from build123d import *

# Parameters (mm, degrees)
F0_R     = 11.1
F1_DEPTH = 7.5
F0_R_2   = 4.25
F2_DEPTH = 7.5
F3_R     = 1.6
F4_DEPTH = 30.501
F5_SIZE  = 0.3
F6_DEPTH = 2.5


with BuildPart() as f1:
    # F0 (on Top) → F1 (new body)
    with BuildSketch(Plane.XY):
        with BuildLine():
            ThreePointArc((0, -14), (9.8994949366, -9.8994949366), (14, 0))
            ThreePointArc((14, 0), (9.8994949366, 9.8994949366), (0, 14))
            ThreePointArc((0, 14), (-14, 0), (0, -14))
        make_face()
        Circle(F0_R, mode=Mode.SUBTRACT)
        with BuildLine():
            ThreePointArc((0, 14), (9.8994949366, 9.8994949366), (14, 0))
            ThreePointArc((14, 0), (9.8994949366, -9.8994949366), (0, -14))
            Line((0, -14), (14, -14))
            Line((14, -14), (14, -22))
            Line((14, -22), (16.5, -22))
            Line((16.5, -22), (16.5, 0))
            Line((16.5, 0), (16.5, 22))
            Line((16.5, 22), (14, 22))
            Line((14, 22), (14, 14))
            Line((14, 14), (0, 14))
        make_face()
    extrude(amount=F1_DEPTH)

    # F0 (on Top) → F2 (join)
    with BuildSketch(Plane.XY):
        with BuildLine():
            ThreePointArc((0, 14), (9.8994949366, 9.8994949366), (14, 0))
            ThreePointArc((14, 0), (9.8994949366, -9.8994949366), (0, -14))
            Line((0, -14), (14, -14))
            Line((14, -14), (14, -22))
            Line((14, -22), (16.5, -22))
            Line((16.5, -22), (16.5, 0))
            Line((16.5, 0), (16.5, 22))
            Line((16.5, 22), (14, 22))
            Line((14, 22), (14, 14))
            Line((14, 14), (0, 14))
        make_face()
        with BuildLine():
            ThreePointArc((0, -14), (9.8994949366, -9.8994949366), (14, 0))
            ThreePointArc((14, 0), (9.8994949366, 9.8994949366), (0, 14))
            ThreePointArc((0, 14), (-14, 0), (0, -14))
        make_face()
        Circle(F0_R, mode=Mode.SUBTRACT)
        Circle(F0_R)
        Circle(F0_R_2, mode=Mode.SUBTRACT)
    extrude(amount=-F2_DEPTH)

    # F3 (on face) → F4 (cut, through all)
    with BuildSketch(Plane.YZ.offset(16.5)):
        with Locations((18, 0)):
            Circle(F3_R)
        with Locations((-18, 0)):
            Circle(F3_R)
    extrude(amount=-F4_DEPTH, mode=Mode.SUBTRACT)

    # F5
    f5_edges = [f1.edges().sort_by_distance(p)[0] for p in [
        (7, -14, -7.5),
        (14, -18, -7.5),
        (15.25, -22, -7.5),
        (16.5, 0, -7.5),
        (15.25, 22, -7.5),
        (14, 18, -7.5),
        (7, 14, -7.5),
        (-14, 0, -7.5),
        (-4.25, 0, -7.5),
    ]]
    chamfer(f5_edges, length=F5_SIZE)

    # F3 (on face) → F6 (join, through all)
    with BuildSketch(Plane.YZ.offset(16.5)):
        with BuildLine():
            ThreePointArc((22, -3), (22.7434164903, -1.5811388301), (23, 0))
            ThreePointArc((23, 0), (22.7434164903, 1.5811388301), (22, 3))
            Line((22, 3), (22, -3))
        make_face()
        with BuildLine():
            Line((22, -3), (22, 3))
            ThreePointArc((22, 3), (13, 0), (22, -3))
        make_face()
        with Locations((18, 0)):
            Circle(F3_R, mode=Mode.SUBTRACT)
        with BuildLine():
            Line((-22, -3), (-22, 3))
            ThreePointArc((-22, 3), (-23, 0), (-22, -3))
        make_face()
    extrude(amount=-F6_DEPTH)


solid = f1.part
Geometry: final body of the model. Coordinates: model frame, mm. A direction names the side the tool comes from. Coordinates: 2 decimals unless noted, no trailing zeros. Loops run counter-clockwise (first coordinate to the right, second up) from the corner with the lowest first, then second, coordinate; pieces in that order, holes last. Notation, with made-up numbers: (48.5, 15) - (93.5, 15) arc R23 cw to (93.5, 40) - close; hole circle Ø10 at (24.25, -10). An arc over 180 degrees is marked (long way). Put each result on its own line as item: value. Start each with the question number.
Q1. Cut plane B-B, the plane z = 3.5. Return loops of the section in (x, y), and give its area (3 significant figures).
Q2. Set-up query: faces 4 (the flat face through (15, -22, 5)), 5 (the flat face through (14, -18, 2)), 6 (the flat face through (5, 0, 0)). Return all of +Z, -Z, +X, -X, +Y, -Y with unobstructed straight access to the full face (end or side cutting, diameter ignored); none if empty.
Q3. Cut plane C-C, the plane y = -18. Return loops of the section in (x, z), and give its area (3 significant figures).
Q4. Cut plane D-D, the plane x = 12. Return loops of the section in (y, z), and give its area (3 significant figures).
Q5. Cut plane A-A, the plane y = 0. Return loops of the section in (x, z), and give its area (3 significant figures).
Q6. Line query: line 1 (Y direction, x = 0, z = -3.25); line 2 (Y direction, x = 0, z = 5.75); line 3 (Z direction, x = 15.4, y = 18). Output: solid intervals per line, ascending.
Q7. Pin query (flat end, axial travel): pin 1 Ø6 at (x, z) = (12.5, 3) entering from +Y; pin 2 Ø1.2 at (x, z) = (15, 5) entering from +Y; pin 3 Ø0.8 at (x, z) = (15, -5) entering from -Y; pin 4 Ø2.5 at (y, z) = (18, 0) entering from +X. Return the tip coordinate at first contact, or that it passes through.
Q8. Pull-direction query (X, two-part tool) for faces 1 (the flat face through (11.3, -1.5, 7.5)), 2 (the cylindrical face through (5.97, 9.36, 3.7)), 3 (the flat face through (16.5, 0, 0)); classes: released by +X, released by -X, zero draft, split by the parting line, or undercut.
Filled sheet:
1. outline: (0, -14) - (14, -14) - (14, -22) - (16.5, -22) - (16.5, 22) - (14, 22) - (14, 14) - (0, 14) arc R14 ccw to start; hole circle Ø22.2 at (0, 0)
1. area: 423 mm²
2. face 4: +Z, +X, -X, -Y
2. face 5: +Z, -Z, -X, -Y
2. face 6: +Z
3. outline: (14, -7.2) - (14.3, -7.5) - (16.2, -7.5) - (16.5, -7.2) - (16.5, -1.6) - (14, -1.6) - close; (14, 1.6) - (16.5, 1.6) - (16.5, 7.5) - (14, 7.5) - close
3. area: 29.4 mm²
4. outline: (-14, -7.2) - (-13.7, -7.5) - (13.7, -7.5) - (14, -7.2) - (14, 7.5) - (-14, 7.5) - close
4. area: 420 mm²
5. outline: (-14, -7.2) - (-13.7, -7.5) - (-4.55, -7.5) - (-4.25, -7.2) - (-4.25, 0) - (-11.1, 0) - (-11.1, 7.5) - (-14, 7.5) - close; (4.25, -7.2) - (4.55, -7.5) - (16.2, -7.5) - (16.5, -7.2) - (16.5, 7.5) - (11.1, 7.5) - (11.1, 0) - (4.25, 0) - close
5. area: 227 mm²
6. line 1: -14 to -4.25, 4.25 to 14
6. line 2: -14 to -11.1, 11.1 to 14
6. line 3: -7.5 to -1.6, 1.6 to 7.5
7. pin 1: y = 22.98
7. pin 2: y = 22
7. pin 3: y = -22
7. pin 4: through
8. face 1: zero draft
8. face 2: undercut
8. face 3: released by +X
